```python
from build123d import *

# Parameters (mm, degrees)
ESQUISSE1_R      = 4.25
EXTRUSION1_DEPTH = 1
ESQUISSE2_R      = 13.5
EXTRUSION2_DEPTH = 36
ESQUISSE3_R      = 4.5
EXTRUSION3_DEPTH = 4.5
ESQUISSE4_R      = 2
EXTRUSION4_DEPTH = 11
ESQUISSE5_R      = 1.5
EXTRUSION5_DEPTH = 4


with BuildPart() as part:
    # Esquisse1 → Extrusion1 (new body)
    with BuildSketch(Plane(origin=(0, 0, 0), x_dir=(1, 0, 0), z_dir=(0, 1, 0))):
        with Locations(Location((0, 0, 0), (0, 0, 270))):
            Circle(ESQUISSE1_R)
    extrude(amount=EXTRUSION1_DEPTH)

    # Esquisse2 → Extrusion2 (add)
    with BuildSketch(Plane(origin=(0, 1, 0), x_dir=(-1, 0, 0), z_dir=(0, 1, 0))):
        with Locations(Location((0, 0, 0), (0, 0, 90))):
            Circle(ESQUISSE2_R)
    extrude(amount=EXTRUSION2_DEPTH)

    # Esquisse3 → Extrusion3 (add)
    with BuildSketch(Plane(origin=(0, 37, 0), x_dir=(-1, 0, 0), z_dir=(0, 1, 0))):
        with Locations(Location((0, 0, 0), (0, 0, 90))):
            Circle(ESQUISSE3_R)
    extrude(amount=EXTRUSION3_DEPTH)

    # Esquisse4 → Extrusion4 (add)
    with BuildSketch(Plane(origin=(0, 41.5, 0), x_dir=(-1, 0, 0), z_dir=(0, 1, 0))):
        with Locations(Location((0, 0, 0), (0, 0, 90))):
            Circle(ESQUISSE4_R)
    extrude(amount=EXTRUSION4_DEPTH)

    # Esquisse5 → Extrusion5 (cut)
    with BuildSketch(Plane(origin=(0, 37, 0), x_dir=(1, 0, 0), z_dir=(0, 1, 0))):
        with Locations(Location((10, 0, 0), (0, 0, 270))):
            Circle(ESQUISSE5_R)
        with Locations(Location((-10, 0, 0), (0, 0, 270))):
            Circle(ESQUISSE5_R)
    extrude(amount=-EXTRUSION5_DEPTH, mode=Mode.SUBTRACT)


solid = part.part
```
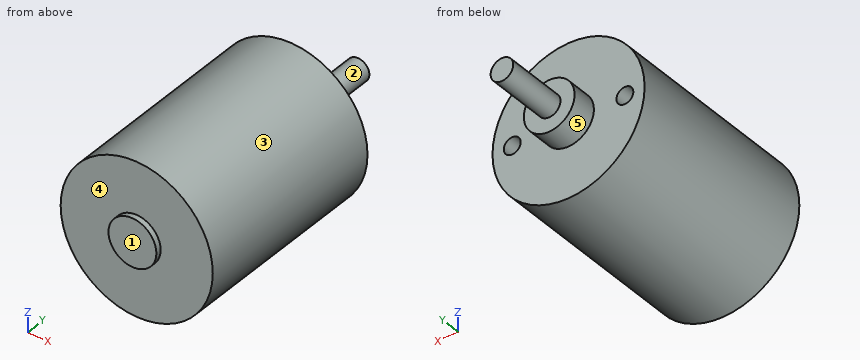
Input: part model. Units: mm. Frame: model coordinates. Face numbers are marked on the shaded views. A direction names the side the tool comes from. Coordinates: 2 decimals unless noted, no trailing zeros. Write each loop counter-clockwise with the first axis right and the second up, starting at its lowest first coordinate (ties: lowest second). Pieces come first, ordered by that corner, then holes.
1) Section A-A on z = 0. Output: boundary loops of the cut face in (x, y), and give its area (3 significant figures).
2) Section C-C on y = 40. Output: boundary loops of the cut face in (x, z).
3) Section D-D on x = -9.25. Output: boundary loops of the cut face in (y, z), and give its area (3 significant figures).
4) Set-up query: the marked faces 3, 4 and 5. Return all of +Z, -Z, +X, -X, +Y, -Y with unobstructed straight access to the full face (end or side cutting, diameter ignored); none if empty.
5) Section B-B on x = 0. Output: boundary loops of the cut face in (y, z), and give its area (4 significant figures).
6) Mould query, pull axis X, two halves, no side actions, for the marked faces 1 and 2. Classes: pulls with the +X half, pulls with the -X half, needs draft (parallel to the pull), parting line crosses it, or undercut.
7) Pin query (flat end, axial travel): pin 1 Ø2.5 at (x, z) = (10, -0.5) entering from +Y; pin 2 Ø5 at (y, z) = (13.5, 8) entering from +X; pin 3 Ø10 at (x, z) = (-8.5, 2) entering from +Y. Return the tip coordinate at first contact, or that it passes through.
8) Material intervals for line 1 along X through (y, z) = (33.9, 0); line 2 along X through (y, z) = (18.5, 0.25); line 3 along Y through (x, z) = (4, -11.75), sorted ascending.
Check result:
1. outline: (-13.5, 1) - (-4.25, 1) - (-4.25, 0) - (4.25, 0) - (4.25, 1) - (13.5, 1) - (13.5, 37) - (11.5, 37) - (11.5, 33) - (8.5, 33) - (8.5, 37) - (4.5, 37) - (4.5, 41.5) - (2, 41.5) - (2, 52.5) - (-2, 52.5) - (-2, 41.5) - (-4.5, 41.5) - (-4.5, 37) - (-8.5, 37) - (-8.5, 33) - (-11.5, 33) - (-11.5, 37) - (-13.5, 37) - close
1. area: 1,040 mm2
2. outline: circle Ø9 at (0, 0)
3. outline: (1, -9.83) - (37, -9.83) - (37, -1.3) - (33, -1.3) - (33, 1.3) - (37, 1.3) - (37, 9.83) - (1, 9.83) - close
3. area: 698 mm2
4. face 3: +Y, -Y
4. face 4: -Y
4. face 5: +Y
5. outline: (0, -4.25) - (1, -4.25) - (1, -13.5) - (37, -13.5) - (37, -4.5) - (41.5, -4.5) - (41.5, -2) - (52.5, -2) - (52.5, 2) - (41.5, 2) - (41.5, 4.5) - (37, 4.5) - (37, 13.5) - (1, 13.5) - (1, 4.25) - (0, 4.25) - close
5. area: 1,065 mm2
6. face 1: needs draft
6. face 2: parting line crosses it
7. pin 1: stops at y = 37
7. pin 2: stops at x = 12.33
7. pin 3: stops at y = 41.5
8. line 1: x = -13.5 to -11.5, -8.5 to 8.5, 11.5 to 13.5
8. line 2: x = -13.5 to 13.5
8. line 3: y = 1 to 37
